The model under review builds one solid part; all positions refer to its coordinate system, in mm. Face numbers are marked on the shaded views. A direction names the side the tool comes from. Coordinates: 2 decimals unless noted, no trailing zeros. Write each loop counter-clockwise with the first axis right and the second up, starting at its lowest first coordinate (ties: lowest second). Pieces come first, ordered by that corner, then holes. Notation, with made-up numbers: (-2, -30.75) - (19, -30.75) arc R22 ccw to (19, -6.75) - close; hole circle Ø8 at (48.25, -15.5). An arc over 180 degrees is marked (long way). Return JSON: item names as keys, results as strings. Group by question number.
(1) Tool access review of the marked faces 1 and 2: name each direction out of +Z, -Z, +X, -X, +Y, -Y from which nothing blocks a thin tool from reaching the whole face with its end or side.
(2) For pin 1 Ø6 at (x, z) = (9, 11) entering from -Y; pin 2 Ø3 at (x, z) = (8.5, 43.5) entering from +Y; pin 3 Ø1.5 at (x, z) = (0.5, 30.5) entering from -Y; pin 4 Ø3 at (y, z) = (-11, 18) entering from +X, all flat-tipped, find the tip position at first contact; note any pin that passes through.
(3) We need section D-D on y = 2.5. State the section outline as (x, z) points.
(4) We need section B-B on z = 41. State the section outline as (x, y) points, then the cut area to 3 significant figures.
(5) To check wall thickness, follow L1, parallel to Z at x = 9, y = 1.8; L2, parallel to X at y = 3.15, z = 41; L3, parallel to Y at x = -0.3, z = 11. State the ranges of each line that lie inside material, in increasing order. Write a range as from..to.
(6) We need section C-C on y = -9. State the section outline as (x, z) points.
(7) We need section A-A on x = 9. State the section outline as (y, z) points.
```python
from build123d import *

# Parameters (mm, degrees)
RESSALTO_EXTRUS_O1_DEPTH = 50
ESBO_O2_R                = 5.15
CORTE_EXTRUS_O1_DEPTH    = 3
ESBO_O3_R                = 5.15
CORTE_EXTRUS_O2_DEPTH    = 3
ESBO_O4_R                = 2
CORTE_EXTRUS_O3_DEPTH    = 10
ESBO_O5_R                = 2
CORTE_EXTRUS_O4_DEPTH    = 10


with BuildPart() as part:
    # Esboço1 → Ressalto-extrusão1 (new body)
    with BuildSketch(Plane.XY):
        Polygon((0, 0), (16, 0), (16, 4), (-4, 4), (-4, -31), (0, -31), align=None)
    extrude(amount=RESSALTO_EXTRUS_O1_DEPTH)

    # Esboço2 → Corte-extrusão1 (cut)
    with BuildSketch(Plane(origin=(0, 4, 0), x_dir=(1, 0, 0), z_dir=(0, 1, 0))):
        with Locations((9, -11)):
            Circle(ESBO_O2_R)
        with Locations((9, -41)):
            Circle(ESBO_O2_R)
    extrude(amount=-CORTE_EXTRUS_O1_DEPTH, mode=Mode.SUBTRACT)

    # Esboço3 → Corte-extrusão2 (cut)
    with BuildSketch(Plane.ZY.offset(4)):
        with Locations((11, -9)):
            Circle(ESBO_O3_R)
        with Locations((41, -9)):
            Circle(ESBO_O3_R)
    extrude(amount=-CORTE_EXTRUS_O2_DEPTH, mode=Mode.SUBTRACT)

    # Esboço4 → Corte-extrusão3 (cut)
    with BuildSketch(Plane.ZY.offset(1)):
        with Locations((11, -9)):
            Circle(ESBO_O4_R)
        with Locations((41, -9)):
            Circle(ESBO_O4_R)
    extrude(amount=-CORTE_EXTRUS_O3_DEPTH, mode=Mode.SUBTRACT)

    # Esboço5 → Corte-extrusão4 (cut)
    with BuildSketch(Plane(origin=(0, 1, 0), x_dir=(1, 0, 0), z_dir=(0, 1, 0))):
        with Locations((9, -11)):
            Circle(ESBO_O5_R)
        with Locations((9, -41)):
            Circle(ESBO_O5_R)
    extrude(amount=-CORTE_EXTRUS_O4_DEPTH, mode=Mode.SUBTRACT)


solid = part.part
```
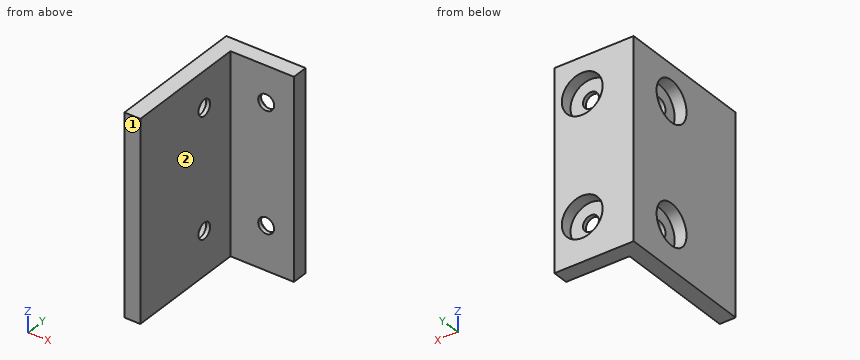
Ans:
{
 "1": {"face 1": "+Z, -Z, +X, -X, -Y", "face 2": "+Z, -Z, +X, -Y"},
 "2": {"pin 1": "y = 0", "pin 2": "y = 1", "pin 3": "y = -31", "pin 4": "x = 0"},
 "3": {"outline": "(-4, 0) - (16, 0) - (16, 50) - (-4, 50) - close; hole circle Ø10.3 at (9, 11); hole circle Ø10.3 at (9, 41)"},
 "4": {"outline": "(-4, -31) - (0, -31) - (0, -11) - (-1, -11) - (-1, -14.15) - (-4, -14.15) - close; (-4, -3.85) - (-1, -3.85) - (-1, -7) - (0, -7) - (0, 0) - (7, 0) - (7, 1) - (3.85, 1) - (3.85, 4) - (-4, 4) - close; (11, 0) - (16, 0) - (16, 4) - (14.15, 4) - (14.15, 1) - (11, 1) - close", "area": "134 mm²"},
 "5": {"L1": "0..5.85, 16.15..35.85, 46.15..50", "L2": "-4..3.85, 14.15..16", "L3": "-31..-11, -7..4"},
 "6": {"outline": "(-4, 0) - (0, 0) - (0, 9) - (-1, 9) - (-1, 5.85) - (-4, 5.85) - close; (-4, 16.15) - (-1, 16.15) - (-1, 13) - (0, 13) - (0, 39) - (-1, 39) - (-1, 35.85) - (-4, 35.85) - close; (-4, 46.15) - (-1, 46.15) - (-1, 43) - (0, 43) - (0, 50) - (-4, 50) - close"},
 "7": {"outline": "(0, 0) - (4, 0) - (4, 5.85) - (1, 5.85) - (1, 9) - (0, 9) - close; (0, 13) - (1, 13) - (1, 16.15) - (4, 16.15) - (4, 35.85) - (1, 35.85) - (1, 39) - (0, 39) - close; (0, 43) - (1, 43) - (1, 46.15) - (4, 46.15) - (4, 50) - (0, 50) - close"}
}
